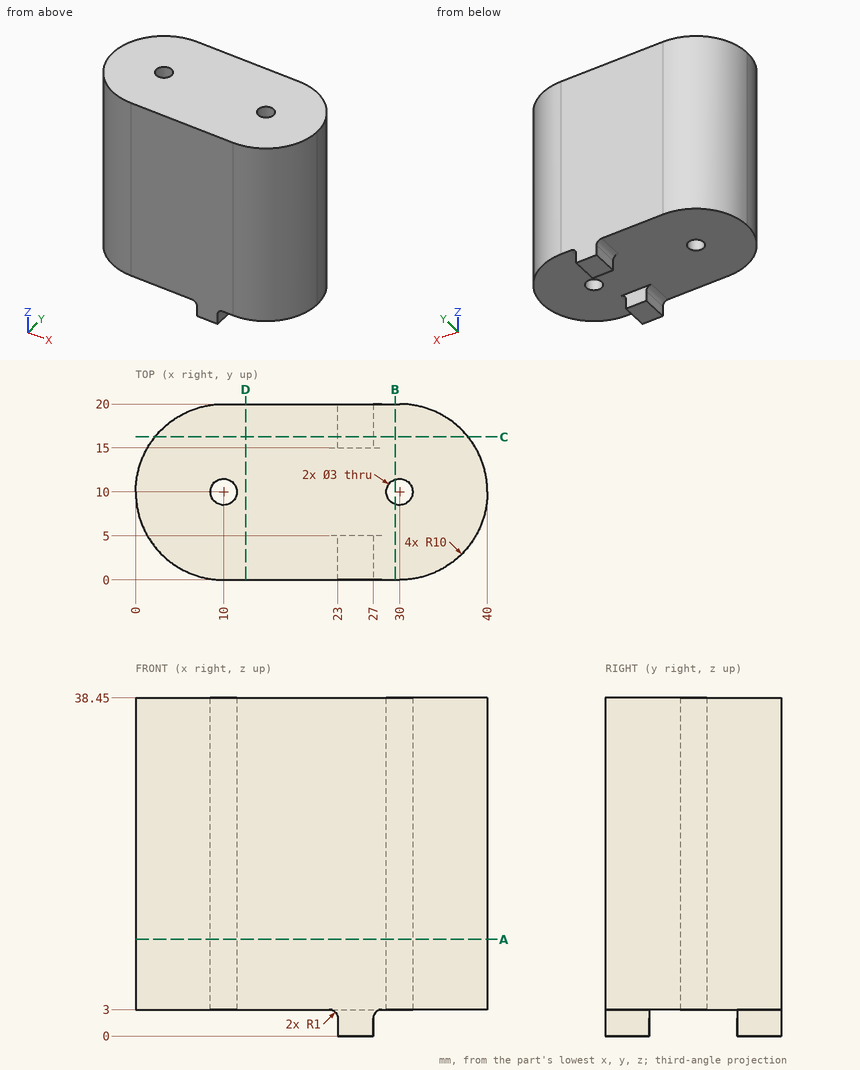
Could you check a few things on this drawing? It's one solid part, dimensions in mm from its lowest x, y, z. Coordinates: 2 decimals unless noted, no trailing zeros. Order: outer loops, then holes, each group sorted by start corner. A loop starts at its lowest first (then second) coordinate and runs counter-clockwise, first axis right, second up. Notation, with made-up numbers: (-20.75, 3) - (-0.75, 3) arc R5 cw to (-0.75, 9) - close; hole circle Ø10 at (3, 59.25). An arc over 180 degrees is marked (long way). One line per question, with ' | ' between items.
(1) Suppose I cut it at D-D on x = 12.5. List the corners of the cut face in (y, z) for me, and give its area (3 significant figures).
Report:
outline: (0, 3) - (20, 3) - (20, 38.45) - (0, 38.45) - close | area: 709 mm2
(2) If I drill on L1, parallel to Y at x = 10, z = 18; L2, parallel to X at y = 9.5, z = 8.5; L3, parallel to Z at x = 33.5, y = 18.5, over which ranges is the centre line in solid material (lowest first)?
Report:
L1: y = 0 to 8.5, 11.5 to 20 | L2: x = 0.01 to 8.59, 11.41 to 28.59, 31.41 to 39.99 | L3: z = 3 to 38.45
(3) Suppose I cut it at A-A on z = 11. State how many separate pieces and enclosed holes the cut face has, and give its area (3 significant figures).
Report:
separate pieces: 1 | enclosed holes: 2 | area: 700 mm2
(4) Suppose I cut it at B-B on x = 29.5. List the corners of the cut face in (y, z) for me.
Report:
outline: (0, 3) - (8.59, 3) - (8.59, 38.45) - (0, 38.45) - close; (11.41, 3) - (20, 3) - (20, 38.45) - (11.41, 38.45) - close
(5) Suppose I cut it at C-C on y = 16.25. List the corners of the cut face in (x, z) for me, and give its area (3 significant figures).
Report:
outline: (2.19, 3) - (22, 3) arc R1 cw to (23, 2) - (23, 0) - (27, 0) - (27, 2) arc R1 cw to (28, 3) - (37.81, 3) - (37.81, 38.45) - (2.19, 38.45) - close | area: 1,270 mm2
(6) Will these pins go through, and if not, where does the flat tip stop? pin 1 (4 mm diameter, centred on x = 31.5, y = 4.5, fed in from -Z); pin 2 (12 mm diameter, centred on x = 19.5, y = 14.5, fed in from -Z); pin 3 (0.6 mm diameter, centred on y = 18.5, z = 1.5, fed in from -X); pin 4 (1 mm diameter, centred on x = 9, z = 29, fed in from -Y).
Report:
pin 1: stops at z = 3 | pin 2: stops at z = 0 | pin 3: stops at x = 23 | pin 4: stops at y = 0.01
